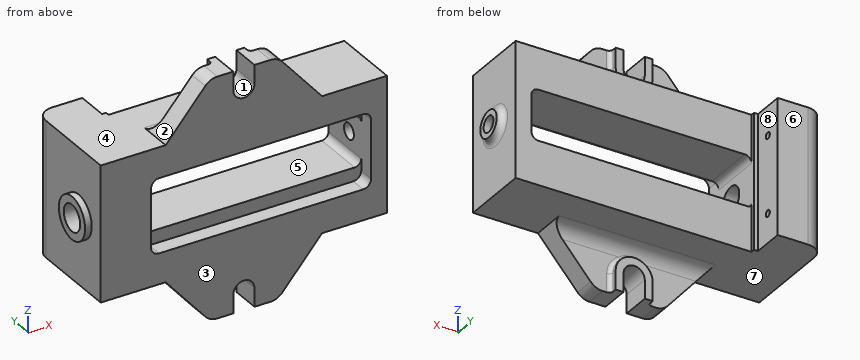
```python
from build123d import *

# Parameters (mm, degrees)
SKETCH1_W             = 216
SKETCH1_H             = 102
EXTRUDE1_DEPTH        = 79
EXTRUDE2_DEPTH        = 169.25278601
FILLET1_R             = 12
EXTRUDE3_DEPTH        = 131.265114286
EXTRUDE4_DEPTH        = 16
EXTRUDE5_DEPTH        = 6
FILLET3_R             = 10
FILLET4_R             = 3
FILLET5_R             = 10
FILLET6_R             = 3
M6_TAPPED_HOLE1_D     = 5
M6_TAPPED_HOLE1_DEPTH = 14
M6_TAPPED_HOLE1_TIP   = 1.502151548
SKETCH13_R            = 10
SKETCH13_R_2          = 6
EXTRUDE7_DEPTH        = 5
EXTRUDE8_REACH        = 248.976
SKETCH14_R            = 6
FILLET7_R             = 5
SKETCH15_R            = 16
EXTRUDE9_DEPTH        = 5
EXTRUDE10_REACH       = 257.767
SKETCH16_R            = 10
EXTRUDE11_DEPTH       = 12


with BuildPart() as part:
    # Sketch1 → Extrude1 (new body)
    with BuildSketch(Plane(origin=(0, 0, 0), x_dir=(1, 0, 0), z_dir=(0, 1, 0))):
        Rectangle(SKETCH1_W, SKETCH1_H)
    extrude(amount=EXTRUDE1_DEPTH)

    # Sketch2 → Extrude2 (cut, through all)
    with BuildSketch(Plane.XY.offset(51)):
        Polygon((-73, 79), (-73, 55), (-70, 55), (-70, 52), (108, 52), (108, 79), align=None)
    extrude(amount=-EXTRUDE2_DEPTH, mode=Mode.SUBTRACT)

    # Fillet1
    fillet1_edges = [part.edges().sort_by_distance(p)[0] for p in [
        (-108, 79, 0),
    ]]
    fillet(fillet1_edges, radius=FILLET1_R)

    # Sketch3 → Extrude3 (cut, through all)
    with BuildSketch(Plane(origin=(0, 52, 0), x_dir=(1, 0, 0), z_dir=(0, 1, 0))):
        with BuildLine():
            Line((-65, -20), (91, -20))
            ThreePointArc((91, -20), (94.535533906, -18.535533906), (96, -15))
            Line((96, -15), (96, 13))
            ThreePointArc((96, 13), (94.535533906, 16.535533906), (91, 18))
            Line((91, 18), (-67, 18))
            ThreePointArc((-67, 18), (-69.121320344, 17.121320344), (-70, 15))
            Line((-70, 15), (-70, -15))
            ThreePointArc((-70, -15), (-68.535533906, -18.535533906), (-65, -20))
        make_face()
    extrude(amount=-EXTRUDE3_DEPTH, mode=Mode.SUBTRACT)

    # Sketch4 → Extrude4 (add)
    with BuildSketch(Plane(origin=(0, 0, 0), x_dir=(1, 0, 0), z_dir=(0, 1, 0))):
        with BuildLine():
            Line((-8, 90), (-20, 90))
            ThreePointArc((-20, 90), (-25.00957212, 88.904319657), (-29.10432929, 85.817364529))
            Line((-29.10432929, 85.817364529), (-59, 51))
            Line((-59, 51), (59, 51))
            Line((59, 51), (29.10432929, 85.817364529))
            ThreePointArc((29.10432929, 85.817364529), (25.00957212, 88.904319657), (20, 90))
            Line((20, 90), (8, 90))
            Line((8, 90), (8, 76))
            ThreePointArc((8, 76), (0, 68), (-8, 76))
            Line((-8, 76), (-8, 90))
        make_face()
        with BuildLine():
            Line((8, -90), (8, -76))
            ThreePointArc((8, -76), (0, -68), (-8, -76))
            Line((-8, -76), (-8, -90))
            Line((-8, -90), (-20, -90))
            ThreePointArc((-20, -90), (-25.00957212, -88.904319657), (-29.10432929, -85.817364529))
            Line((-29.10432929, -85.817364529), (-59, -51))
            Line((-59, -51), (59, -51))
            Line((59, -51), (29.10432929, -85.817364529))
            ThreePointArc((29.10432929, -85.817364529), (25.00957212, -88.904319657), (20, -90))
            Line((20, -90), (8, -90))
        make_face()
    extrude(amount=EXTRUDE4_DEPTH)

    # Sketch5 → Extrude5 (add)
    with BuildSketch(Plane(origin=(0, 16, 0), x_dir=(1, 0, 0), z_dir=(0, 1, 0))):
        with BuildLine():
            Line((-14, -90), (-14, -76))
            ThreePointArc((-14, -76), (0, -62), (14, -76))
            Line((14, -76), (14, -90))
            Line((14, -90), (8, -90))
            Line((8, -90), (8, -76))
            ThreePointArc((8, -76), (0, -68), (-8, -76))
            Line((-8, -76), (-8, -90))
            Line((-8, -90), (-14, -90))
        make_face()
        with BuildLine():
            Line((14, 90), (14, 76))
            ThreePointArc((14, 76), (0, 62), (-14, 76))
            Line((-14, 76), (-14, 90))
            Line((-14, 90), (-8, 90))
            Line((-8, 90), (-8, 76))
            ThreePointArc((-8, 76), (0, 68), (8, 76))
            Line((8, 76), (8, 90))
            Line((8, 90), (14, 90))
        make_face()
    extrude(amount=EXTRUDE5_DEPTH)

    # Fillet3
    fillet3_edges = [part.edges().sort_by_distance(p)[0] for p in [
        (0, 16, 51),
    ]]
    fillet(fillet3_edges, radius=FILLET3_R)

    # Fillet4
    fillet4_edges = [part.edges().sort_by_distance(p)[0] for p in [
        (14, 16, 83),
        (0, 16, 62),
        (-14, 16, 83),
    ]]
    fillet(fillet4_edges, radius=FILLET4_R)

    # Fillet5
    fillet5_edges = [part.edges().sort_by_distance(p)[0] for p in [
        (0, 16, -51),
    ]]
    fillet(fillet5_edges, radius=FILLET5_R)

    # Fillet6
    fillet6_edges = [part.edges().sort_by_distance(p)[0] for p in [
        (0, 16, -62),
        (14, 16, -83),
        (-14, 16, -83),
    ]]
    fillet(fillet6_edges, radius=FILLET6_R)

    # M6 Tapped Hole1
    with Locations(Plane(origin=(-73, 67, 29), x_dir=(0, 0, 1), z_dir=(1, 0, 0))):
        with Locations((0, 0), (-58, 0)):
            Hole(M6_TAPPED_HOLE1_D / 2, depth=M6_TAPPED_HOLE1_DEPTH)
            with Locations((0, 0, -(M6_TAPPED_HOLE1_DEPTH + M6_TAPPED_HOLE1_TIP / 2))):  # 118° drill point
                Cone(0, M6_TAPPED_HOLE1_D / 2, M6_TAPPED_HOLE1_TIP, mode=Mode.SUBTRACT)

    # Sketch13 → Extrude7 (add)
    with BuildSketch(Plane(origin=(108, 0, 0), x_dir=(0, 0, -1), z_dir=(1, 0, 0))):
        with Locations(Location((0, 27, 0), (0, 0, 180))):
            Circle(SKETCH13_R)
        with Locations((0, 27)):
            Circle(SKETCH13_R_2, mode=Mode.SUBTRACT)
    extrude(amount=EXTRUDE7_DEPTH)

    # Sketch14 → Extrude8 (cut, up to next)
    with BuildSketch(Plane(origin=(108, 0, 0), x_dir=(0, 0, -1), z_dir=(1, 0, 0)), mode=Mode.PRIVATE) as extrude8_sk1:
        with Locations((0, 27)):
            Circle(SKETCH14_R)
    extrude8_tool1 = extrude(extrude8_sk1.sketch, amount=-EXTRUDE8_REACH, mode=Mode.PRIVATE) & part.part
    add(extrude8_tool1.solids().sort_by_distance((108, 27, 0))[0], mode=Mode.SUBTRACT)

    # Fillet7
    fillet7_edges = [part.edges().sort_by_distance(p)[0] for p in [
        (108, 27, -10),
    ]]
    fillet(fillet7_edges, radius=FILLET7_R - 0.0001)  # a hair under: the kernel refuses the full size

    # Sketch15 → Extrude9 (add)
    with BuildSketch(Plane.ZY.offset(108)):
        with Locations(Location((0, 27, 0), (0, 0, 180))):
            Circle(SKETCH15_R)
    extrude(amount=EXTRUDE9_DEPTH)

    # Sketch16 → Extrude10 (cut, up to next)
    with BuildSketch(Plane.ZY.offset(113), mode=Mode.PRIVATE) as extrude10_sk1:
        with Locations((0, 27)):
            Circle(SKETCH16_R)
    extrude10_tool1 = extrude(extrude10_sk1.sketch, amount=-EXTRUDE10_REACH, mode=Mode.PRIVATE) & part.part
    add(extrude10_tool1.solids().sort_by_distance((-113, 27, 0))[0], mode=Mode.SUBTRACT)

    # Sketch17 → Extrude11 (cut)
    with BuildSketch(Plane.XZ):
        with BuildLine():
            Line((-64, -28), (90, -28))
            ThreePointArc((90, -28), (94.242640687, -26.242640687), (96, -22))
            Line((96, -22), (96, 22))
            ThreePointArc((96, 22), (94.242640687, 26.242640687), (90, 28))
            Line((90, 28), (-64, 28))
            ThreePointArc((-64, 28), (-68.242640687, 26.242640687), (-70, 22))
            Line((-70, 22), (-70, -22))
            ThreePointArc((-70, -22), (-68.242640687, -26.242640687), (-64, -28))
        make_face()
    extrude(amount=-EXTRUDE11_DEPTH, mode=Mode.SUBTRACT)


solid = part.part
```
Model file for the job. Use its own axes, mm. Face numbers are marked on the shaded views. A direction names the side the tool comes from. Give positions to 0.01 mm unless a question says otherwise; leave off trailing zeros. Write each loop counter-clockwise with the first axis right and the second up, starting at its lowest first coordinate (ties: lowest second). Pieces come first, ordered by that corner, then holes. Notation, with made-up numbers: (-24, 69.5) -> (31, 69.5) arc R5 ccw to (31, 78.5) -> close; hole circle Ø7 at (-12, -16). An arc over 180 degrees is marked (long way). Use CSV: the item, a comma, the result in double quotes. Start each with the question number.
1) Cut at B-B on x = -42. List the corners of the cut face in (y, z).
2) Cut at A-A on z = 0. Count the separate pieces of the cut face and the enclosed holes in it, plus the area to 3 significant figures.
3) Drill centre lines: L1, parallel to Y at x = -82, z = 29; L2, parallel to Z at x = -46, y = 36; L3, parallel to X at y = 4.5, z = 22. Where is each one in solid material? Low to high.
4) Two-plate mould, pull along X, no slides. Class the marked faces 1, 2 and 3: released by +X, released by -X, zero draft, split by the parting line, or undercut.
5) Cut at D-D on y = 58.5. List the corners of the cut face in (x, z).
6) Tool access for the marked faces 4, 5, 6, 7 and 8: list every direction of +Z, -Z, +X, -X, +Y, -Y with a clear straight run to the whole face (end or side of a thin tool).
7) Pin check, flat tips, straight feed: P1, Ø19, axis at y = 27, z = 0, coming from the +X side; P2, Ø3, axis at y = 34, z = 18, coming from the -X side; P3, Ø6, axis at x = 80, y = 52.5, coming from the -Z side; P4, Ø1, axis at x = 75.5, y = 47.5, coming from the +Z side. Stop position of each tip, or through.
Final values:
1,outline,"(0, -70.8) -> (16, -70.8) -> (16, -61) arc R10 cw to (26, -51) -> (52, -51) -> (52, -18) -> (12, -18) -> (12, -28) -> (0, -28) -> close; (0, 28) -> (12, 28) -> (12, 20) -> (52, 20) -> (52, 51) -> (26, 51) arc R10 cw to (16, 61) -> (16, 70.8) -> (0, 70.8) -> close"
2,separate pieces,"4"
2,enclosed holes,"0"
2,area,"2,730 mm2"
3,L1,"y = 0 to 64.5, 69.5 to 79"
3,L2,"z = -51 to -18, 20 to 51"
3,L3,"x = -108 to -70, 96 to 108"
4,face 1,"undercut"
4,face 2,"released by -X"
4,face 3,"zero draft"
5,outline,"(-108, -51) -> (-73, -51) -> (-73, 51) -> (-108, 51) -> close"
6,face 4,"+Z, +Y"
6,face 5,"+Y, -Y"
6,face 6,"+Z, -Z, +X, -X, +Y"
6,face 7,"-Z, +Y"
6,face 8,"+Z, -Z, +X, +Y"
7,P1,"stops at x = 113"
7,P2,"stops at x = -108"
7,P3,"stops at z = -51"
7,P4,"stops at z = 51"
